from build123d import *

# Parameters (mm, degrees)
F1_DEPTH = 14.0906665474
F3_D     = 45.72
F4_R     = 6.858
F5_R     = 6.858


with BuildPart() as f1:
    # F0 (on Front) → F1 (new body)
    with BuildSketch(Plane.XZ):
        with BuildLine():
            ThreePointArc((26.423855446, -8.2792220637), (27.3665356573, -4.201095127), (27.6831785203, -0.0274273648))
            ThreePointArc((27.6831785203, -0.0274273648), (27.364375928, 4.1603676932), (26.4153157441, 8.251644671))
            Line((26.4153157441, 8.251644671), (-26.3786924152, 8.251644671))
            ThreePointArc((-26.3786924152, 8.251644671), (-27.6465515, -0.0131359372), (-26.3872321171, -8.2792220637))
            Line((-26.3872321171, -8.2792220637), (26.423855446, -8.2792220637))
        make_face()
        with BuildLine():
            ThreePointArc((26.4153157441, 8.251644671), (27.364375928, 4.1603676932), (27.6831785203, -0.0274273648))
            ThreePointArc((27.6831785203, -0.0274273648), (27.3665356573, -4.201095127), (26.423855446, -8.2792220637))
            Line((26.423855446, -8.2792220637), (32.2108827531, -8.2792220637))
            Line((32.2108827531, -8.2792220637), (32.2108827531, 8.251644671))
            Line((32.2108827531, 8.251644671), (26.4153157441, 8.251644671))
        make_face()
        with BuildLine():
            Line((-26.3786924152, 8.251644671), (26.4153157441, 8.251644671))
            ThreePointArc((26.4153157441, 8.251644671), (0.0183116645, 27.6374394911), (-26.3786924152, 8.251644671))
        make_face()
        with BuildLine():
            ThreePointArc((-26.3872321171, -8.2792220637), (0.0183116645, -27.6922942207), (26.423855446, -8.2792220637))
            Line((26.423855446, -8.2792220637), (-26.3872321171, -8.2792220637))
        make_face()
        with BuildLine():
            ThreePointArc((-26.3872321171, -8.2792220637), (-27.6465515, -0.0131359372), (-26.3786924152, 8.251644671))
            Line((-26.3786924152, 8.251644671), (-31.9677777588, 8.251644671))
            Line((-31.9677777588, 8.251644671), (-31.9677777588, -8.2792220637))
            Line((-31.9677777588, -8.2792220637), (-26.3872321171, -8.2792220637))
        make_face()
    extrude(amount=F1_DEPTH)

    # F3 (through all)
    with Locations(Plane(origin=(0, 0, 0), x_dir=(1, 0, 0), z_dir=(0, 1, 0))):
        with Locations((0, 0)):
            Hole(F3_D / 2)

    # F4
    f4_edges = [f1.edges().sort_by_distance(p)[0] for p in [
        (29.317369, -14.090667, -8.279222),
        (29.317369, 0, -8.279222),
        (29.313099, -14.090667, 8.251645),
        (29.313099, 0, 8.251645),
    ]]
    fillet(f4_edges, radius=F4_R)

    # F5
    f5_edges = [f1.edges().sort_by_distance(p)[0] for p in [
        (-29.177505, -14.090667, -8.279222),
        (-29.173235, -14.090667, 8.251645),
        (-29.173235, 0, 8.251645),
        (-29.177505, 0, -8.279222),
    ]]
    fillet(f5_edges, radius=F5_R)


solid = f1.part
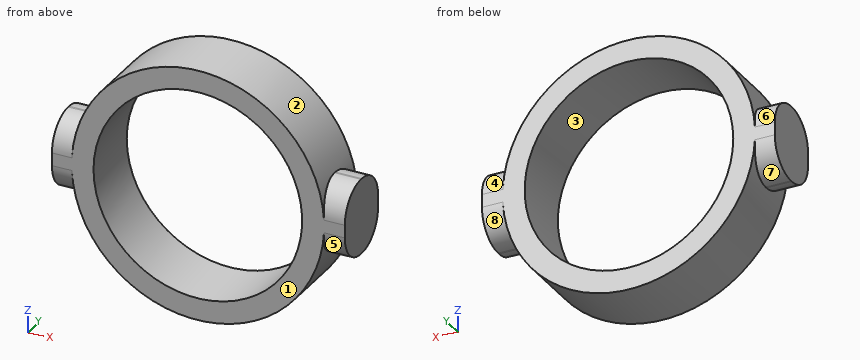
Read the model definition and answer for the solid it produces. Units are mm, in the model's axes. Face numbers are marked on the shaded views. A direction names the side the tool comes from. Round coordinates to 2 decimals unless told otherwise and drop trailing zeros. Write each loop counter-clockwise with the first axis right and the second up, starting at its lowest first coordinate (ties: lowest second). Pieces come first, ordered by that corner, then holes. Notation, with made-up numbers: (-22.75, 27) - (27.25, 27) arc R17 ccw to (27.25, 43) - close; hole circle Ø6 at (-4, 47.5). An arc over 180 degrees is marked (long way). One line per question, with ' | ' between items. Start each with the question number.
1. Section D-D (z = 6) is taken. Determine the outline of the cut face in (x, y).
2. For the marked faces 4, 5, 6, 7 and 8, determine the directions among +Z, -Z, +X, -X, +Y, -Y from which every point of the face is accessible in a straight line to the end or side of a thin tool.
3. Each of these flat-tipped pins is pushed along its axis until it touches: pin 1 (3 mm diameter, centred on x = 23.5, y = -2, fed in from +Z); pin 2 (1.5 mm diameter, centred on x = -3.5, y = -3, fed in from -Z); pin 3 (2 mm diameter, centred on y = -3.5, z = -22, fed in from -X). Where does it stop, or does it pass through?
4. Section C-C (y = -8.5) is taken. Determine the outline of the cut face in (x, z), and give its area (3 significant figures).
5. Section B-B (x = 0) is taken. Determine the outline of the cut face in (y, z), and give its area (3 significant figures).
6. Find the intervals of material crossed by probe 1 along Z at (x, y) = (0, -8); probe 2 along Z at (x, y) = (18.5, -7); probe 3 along X at (y, z) = (-8.5, 14), in increasing order. Write a range as [from, to].
7. Section A-A (z = 0) is taken. Determine the outline of the cut face in (x, y).
8. For a pull along X with two mould halves and no side action, classify the marked faces 1, 2 and 3 as +X half, -X half, draft (parallel to the pull), parting line (faces both ways), or undercut.
Filled in:
1) outline: (-31.97, -12.31) - (-26.98, -12.31) - (-26.98, -14.09) - (-22.06, -14.09) - (-22.06, 0) - (-26.98, 0) - (-26.98, -1.78) - (-31.97, -1.78) - close; (22.06, -14.09) - (27.02, -14.09) - (27.02, -12.31) - (32.21, -12.31) - (32.21, -1.78) - (27.02, -1.78) - (27.02, 0) - (22.06, 0) - close
2) face 4: +Z, +X, +Y | face 5: -Z, +X, -Y | face 6: +Z, -X, +Y | face 7: -Z, -X, +Y | face 8: -Z, +X, +Y
3) pin 1: z = 16.77 | pin 2: z = -27.55 | pin 3: x = -18.02
4) outline: (-31.97, -8.16) - (-26.42, -8.16) arc R27.66 ccw to (26.46, -8.16) - (32.21, -8.16) - (32.21, 8.13) - (26.45, 8.13) arc R27.66 ccw to (-26.42, 8.13) - (-31.97, 8.13) - close; hole circle Ø45.72 at (0, 0) | area: 920 mm²
5) outline: (-14.09, -27.69) - (0, -27.69) - (0, -22.86) - (-14.09, -22.86) - close; (-14.09, 22.86) - (0, 22.86) - (0, 27.64) - (-14.09, 27.64) - close | area: 135 mm²
6) probe 1: [-27.69, -22.86], [22.86, 27.64] | probe 2: [-20.61, -13.43], [13.43, 20.56] | probe 3: [-23.83, -18.07], [18.07, 23.86]
7) outline: (-31.97, -14.09) - (-22.86, -14.09) - (-22.86, 0) - (-31.97, 0) - close; (22.86, -14.09) - (32.21, -14.09) - (32.21, 0) - (22.86, 0) - close
8) face 1: draft | face 2: parting line | face 3: undercut
